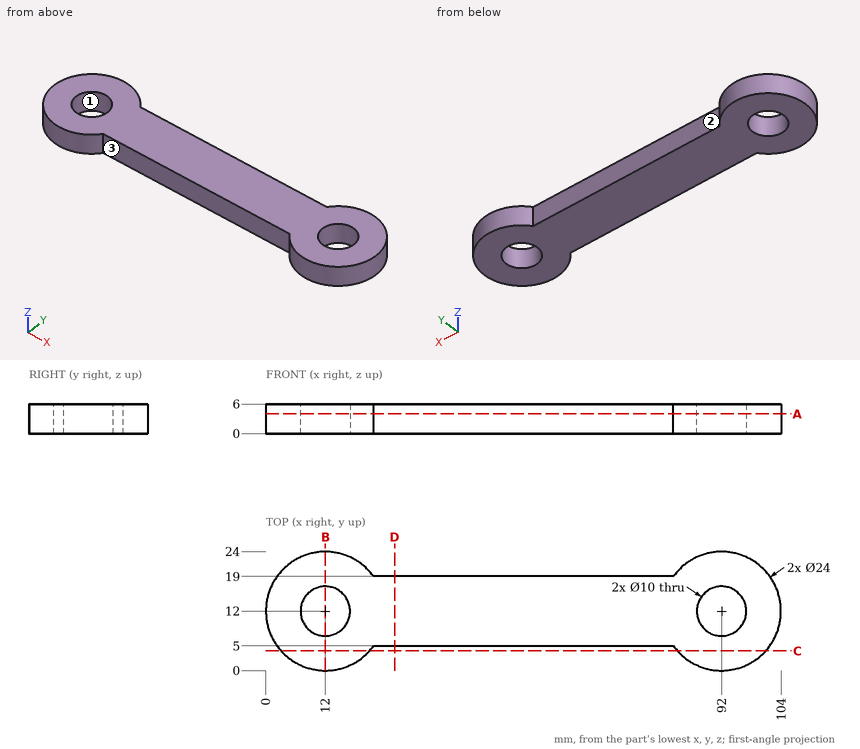
Print and shaded views of the part. All mm, measured from the part's lowest x, y and z. A direction names the side the tool comes from. Coordinates: 2 decimals unless noted, no trailing zeros. Write each loop counter-clockwise with the first axis right and the second up, starting at its lowest first coordinate (ties: lowest second). Pieces come first, ordered by that corner, then holes. Notation, with made-up numbers: M 10.5,70.25 L 18.5,70.25 A15 cw 18.5,89.25 Z; hole C 18,87 d3. An arc over 180 degrees is marked long. Return JSON: item names as keys, results as strings.
1. Flat gauge pins, fed straight in: pin 1 Ø4 at (x, y) = (74.5, 4) entering from -Z; pin 2 Ø1 at (x, z) = (57, 2) entering from +Y; pin 3 Ø1 at (y, z) = (10.5, 5.5) entering from -X; pin 4 Ø3 at (x, z) = (59.5, 4) entering from -Y. Where does each tip first touch, or does it go through?
Determined:
{"pin 1": "z = 0", "pin 2": "y = 19", "pin 3": "x = 0.04", "pin 4": "y = 5"}
2. Saw through at B-B, the plane x = 12. Write the cut outline in (y, z), then the cut area to 3 significant figures.
Determined:
{"outline": "M 0,0 L 7,0 L 7,6 L 0,6 Z; M 17,0 L 24,0 L 24,6 L 17,6 Z", "area": "84.0 mm²"}
3. Saw through at D-D, the plane x = 26. Write the cut outline in (y, z).
Determined:
{"outline": "M 5,0 L 19,0 L 19,6 L 5,6 Z"}
4. Probe L1, parallel to Y at x = 92, z = 2.6; L2, parallel to X at y = 11.5, z = 3.35; L3, parallel to X at y = 15.5, z = 5.4. List the from-to ranges inside material, lowest first.
Determined:
{"L1": "0 to 7, 17 to 24", "L2": "0.01 to 7.03, 16.97 to 87.03, 96.97 to 103.99", "L3": "0.52 to 8.43, 15.57 to 88.43, 95.57 to 103.48"}
5. 3-axis set-ups, long thin cutter, end or side, ignore diameter. For the marked faces 1, 2 and 3: which of +Z, -Z, +X, -X, +Y, -Y reach the whole face in a straight line?
Determined:
{"face 1": "+Z, -Z", "face 2": "+Z, -Z, +Y", "face 3": "+Z, -Z, -Y"}
6. Saw through at A-A, the plane z = 4. Write the cut outline in (x, y).
Determined:
{"outline": "M 21.75,5 L 82.25,5 A12 ccw long 82.25,19 L 21.75,19 A12 ccw long Z; hole C 12,12 d10; hole C 92,12 d10"}
7. Saw through at C-C, the plane y = 4. Write the cut outline in (x, z), then the cut area to 3 significant figures.
Determined:
{"outline": "M 3.06,0 L 20.94,0 L 20.94,6 L 3.06,6 Z; M 83.06,0 L 100.94,0 L 100.94,6 L 83.06,6 Z", "area": "215 mm²"}
